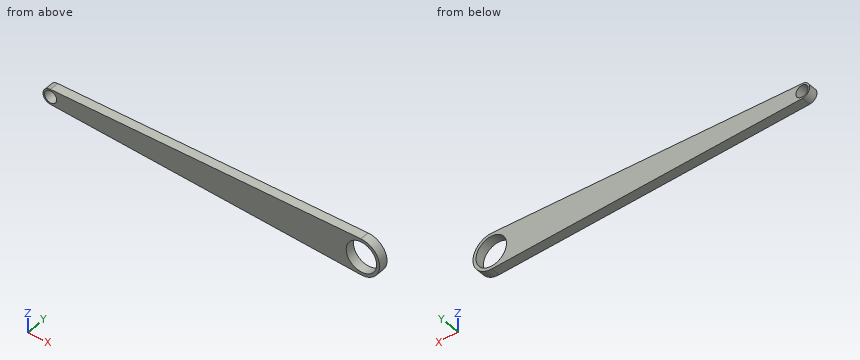
```python
from build123d import *

# Parameters (mm, degrees)
BOSS_EXTRUDE1_DEPTH = 0.75
CUT_EXTRUDE1_REACH  = 54.358
SKETCH3_R           = 2.5
SKETCH3_R_2         = 1


with BuildPart() as part:
    # Sketch2 → Boss-Extrude1 (new, symmetric)
    with BuildSketch(Plane(origin=(0, 0, 0), x_dir=(1, 0, 0), z_dir=(0, 1, 0))):
        with BuildLine():
            Line((-51.042892157, 1.249263888), (-0.102941176, 2.998233332))
            ThreePointArc((-0.102941176, 2.998233332), (3, 0), (-0.102941176, -2.998233332))
            Line((-0.102941176, -2.998233332), (-51.042892157, -1.249263888))
            ThreePointArc((-51.042892157, -1.249263888), (-52.25, 0), (-51.042892157, 1.249263888))
        make_face()
    extrude(amount=BOSS_EXTRUDE1_DEPTH, both=True)

    # Sketch3 → Cut-Extrude1 (cut, up to next)
    with BuildSketch(Plane(origin=(0, 0.75, 0), x_dir=(1, 0, 0), z_dir=(0, 1, 0)), mode=Mode.PRIVATE) as cut_extrude1_sk1:
        with Locations(Location((0, 0, 0), (0, 0, 270))):
            Circle(SKETCH3_R)
    cut_extrude1_tool1 = extrude(cut_extrude1_sk1.sketch, amount=-CUT_EXTRUDE1_REACH, mode=Mode.PRIVATE) & part.part
    # Sketch3 → Cut-Extrude1 (cut, up to next)
    with BuildSketch(Plane(origin=(0, 0.75, 0), x_dir=(1, 0, 0), z_dir=(0, 1, 0)), mode=Mode.PRIVATE) as cut_extrude1_sk2:
        with Locations(Location((-51, 0, 0), (0, 0, 270))):
            Circle(SKETCH3_R_2)
    cut_extrude1_tool2 = extrude(cut_extrude1_sk2.sketch, amount=-CUT_EXTRUDE1_REACH, mode=Mode.PRIVATE) & part.part
    add(cut_extrude1_tool1.solids().sort_by_distance((0, 0.75, 0))[0], mode=Mode.SUBTRACT)
    add(cut_extrude1_tool2.solids().sort_by_distance((-51, 0.75, 0))[0], mode=Mode.SUBTRACT)


solid = part.part
```
Here's how the part is built. I have some questions about the finished solid (model axes, mm). Coordinates: 2 decimals unless noted, no trailing zeros. Order: outer loops, then holes, each group sorted by start corner. A loop starts at its lowest first (then second) coordinate and runs counter-clockwise, first axis right, second up. Notation, with made-up numbers: (-33, 43) - (-25, 43) arc R21 ccw to (-25, 80) - close; hole circle Ø2 at (43, 40). An arc over 180 degrees is marked (long way). One line per question, with ' | ' between items.
(1) If I drill on L1, parallel to X at y = -0.5, z = 0.1; L2, parallel to X at y = 0.25, z = 0.8; L3, parallel to Z at x = -9, y = 0.55, over which ranges is the centre line in solid material (lowest first)?
Report:
L1: x = -52.25 to -51.99, -50.01 to -2.5, 2.5 to 3 | L2: x = -51.96 to -51.6, -50.4 to -2.37, 2.37 to 2.89 | L3: z = -2.69 to 2.69
(2) Suppose I cut it at B-B on z = 0. List the corners of the cut face in (x, y) for me, and give its area (3 significant figures).
Report:
outline: (-52.25, -0.75) - (-52, -0.75) - (-52, 0.75) - (-52.25, 0.75) - close; (-50, -0.75) - (-2.5, -0.75) - (-2.5, 0.75) - (-50, 0.75) - close; (2.5, -0.75) - (3, -0.75) - (3, 0.75) - (2.5, 0.75) - close | area: 72.4 mm2
(3) Will this pin go through, and if not, where does the flat tip stop? pin 1 (1.6 mm diameter, centred on x = -51, z = 0, fed in from -Y).
Report:
pin 1: passes through
(4) Suppose I cut it at C-C on x = -1. List the corners of the cut face in (y, z) for me, and give its area (3 significant figures).
Report:
outline: (-0.75, -2.97) - (0.75, -2.97) - (0.75, -2.29) - (-0.75, -2.29) - close; (-0.75, 2.29) - (0.75, 2.29) - (0.75, 2.97) - (-0.75, 2.97) - close | area: 2.03 mm2
(5) Suppose I cut it at A-A on y = 0. List the corners of the cut face in (x, z) for me.
Report:
outline: (-51.04, -1.25) - (-0.1, -3) arc R3 ccw (long way) to (-0.1, 3) - (-51.04, 1.25) arc R1.25 ccw to start; hole circle Ø2 at (-51, 0); hole circle Ø5 at (0, 0)
(6) Suppose I cut it at D-D on x = -11. List the corners of the cut face in (y, z) for me, and give its area (3 significant figures).
Report:
outline: (-0.75, -2.62) - (0.75, -2.62) - (0.75, 2.62) - (-0.75, 2.62) - close | area: 7.87 mm2
